```python
from build123d import *

# Parameters (mm, degrees)
F0_W     = 584.2
F0_H     = 74.632816
F1_DEPTH = 19.05


with BuildPart() as f1:
    # F0 (on Front) → F1 (new body)
    with BuildSketch(Plane.XZ):
        Polygon((0, 46.99), (0, 0), (584.2, 0), (584.2, 46.99), (603.25, 46.99), (603.25, 97.79), (584.2, 97.79), (584.2, 250.19), (603.25, 250.19), (603.25, 300.99), (584.2, 300.99), (584.2, 347.98), (0, 347.98), (0, 300.99), (-19.05, 300.99), (-19.05, 250.19), (0, 250.19), (0, 97.79), (-19.05, 97.79), (-19.05, 46.99), align=None)
        with Locations((292.1, 385.296408)):
            Rectangle(F0_W, F0_H)
    extrude(amount=F1_DEPTH)


solid = f1.part
```
For this review, take the finished solid that the model builds, in its own axes (mm). A direction names the side the tool comes from. Give positions to 0.01 mm unless a question says otherwise; leave off trailing zeros. Loops run counter-clockwise (first coordinate to the right, second up) from the corner with the lowest first, then second, coordinate; pieces in that order, holes last. Notation, with made-up numbers: M 34,19 L 73,19 A5 cw 73,26 Z; hole C -5,29 d2. An arc over 180 degrees is marked long. One line per item, written item: value. Start each with the question number.
Q1. Machinability: for faces 5 (the face through (584.2, -9, 361)), 6 (the face through (594, -9, 46.99)), 7 (the face through (584.2, -9, 173)), 8 (the face through (0, -9, 175)), which of the approach directions +Z, -Z, +X, -X, +Y, -Y give a long, thin tool a straight path to every point of the face, cutting with its end or side? Answer none if there is none.
Q2. Add section A-A (y = -12.5). Give the boundary of the cut face in (x, z), and give its area (3 significant figures).
Q3. Clearance check with flat-ended pins moving along their axes: pin 1 Ø4 at (y, z) = (-13.5, 349) entering from -X; pin 2 Ø5.5 at (y, z) = (-6.5, 16.5) entering from +X; pin 3 Ø9.5 at (x, y) = (-11, -13) entering from +Z; pin 4 Ø12 at (x, z) = (209.5, 322) entering from +Y. State where each tip first meets the part, or that it passes through.
Q4. Add section B-B (z = 131.5). Give the boundary of the cut face in (x, y).
Q5. Draft analysis for pull direction Z (two halves, no side actions). For faces 1 (the face through (594, -9, 97.79)), 2 (the face through (-9, -9, 97.79)), 3 (the face through (-10, -9, 46.99)), 4 (the face through (-9, -9, 300.99)), state which applies: released by +Z, released by -Z, zero draft, split by the parting line, or undercut.
Q6. For L1, parallel to X at y = -3.5, z = 157, list the stretches that pass through material, from the lowest coordinate up.
Reply:
1. face 5: +Z, +X, +Y, -Y
1. face 6: -Z, +X, +Y, -Y
1. face 7: +X, +Y, -Y
1. face 8: -X, +Y, -Y
2. outline: M -19.05,46.99 L 0,46.99 L 0,0 L 584.2,0 L 584.2,46.99 L 603.25,46.99 L 603.25,97.79 L 584.2,97.79 L 584.2,250.19 L 603.25,250.19 L 603.25,300.99 L 584.2,300.99 L 584.2,422.61 L 0,422.61 L 0,300.99 L -19.05,300.99 L -19.05,250.19 L 0,250.19 L 0,97.79 L -19.05,97.79 Z
2. area: 251,000 mm²
3. pin 1: x = 0
3. pin 2: x = 584.2
3. pin 3: z = 300.99
3. pin 4: y = 0
4. outline: M 0,-19.05 L 584.2,-19.05 L 584.2,0 L 0,0 Z
5. face 1: undercut
5. face 2: undercut
5. face 3: released by -Z
5. face 4: released by +Z
6. L1: 0 to 584.2
